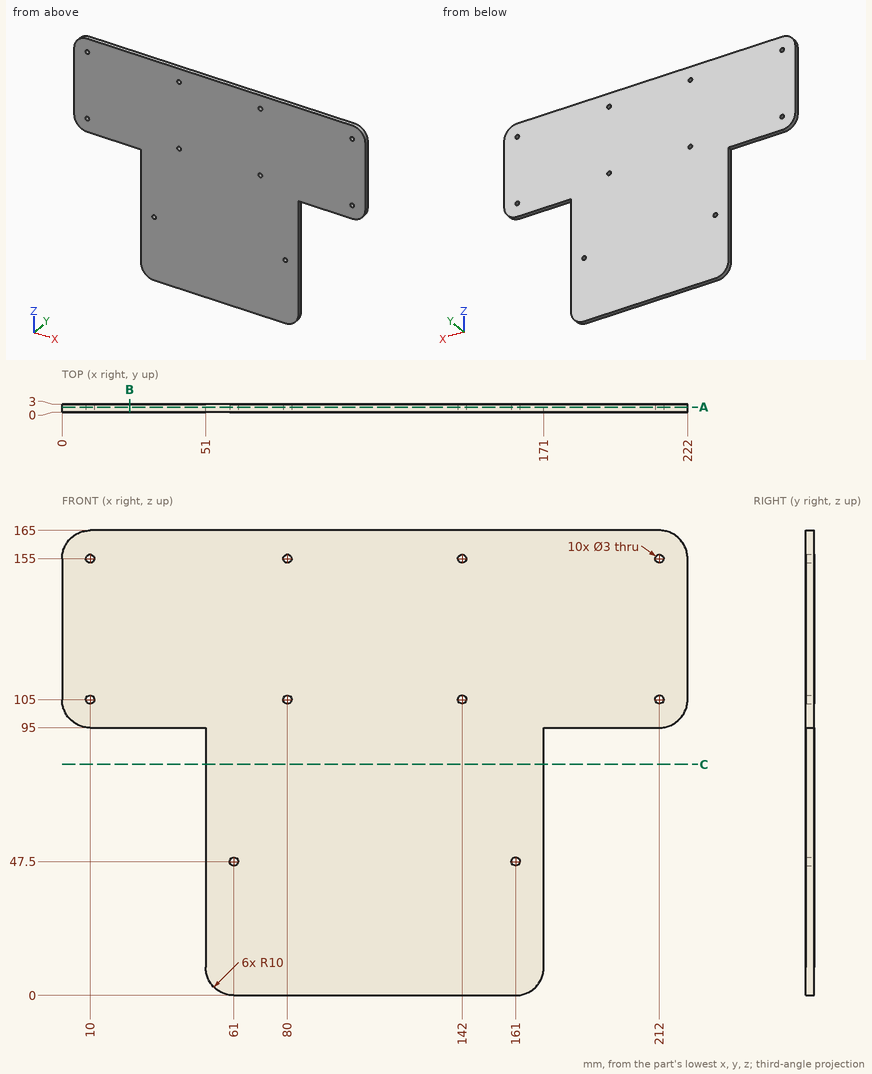
Input: dimensioned drawing with shaded views. Units: mm. Origin: part minimum x, y, z. Give positions to 0.01 mm unless a question says otherwise; leave off trailing zeros. Order: outer loops, then holes, each group sorted by start corner. A loop starts at its lowest first (then second) coordinate and runs counter-clockwise, first axis right, second up. Notation, with made-up numbers: (65, 45) -> (94, 45) arc R24 ccw to (94, 66) -> close; hole circle Ø4 at (22.5, -13.5). An arc over 180 degrees is marked (long way). Use a Markdown table: item, result.
1) Section query A-A, the plane y = 1.9. Count the separate pieces of the cut face and the enclosed holes in it, then the cut area to 3 significant figures.
Answer list:
| item | result |
|---|---|
| separate pieces | 1 |
| enclosed holes | 10 |
| area | 26,700 mm² |
2) Section query B-B, the plane x = 24. Return the cut outline in (y, z).
Answer list:
| item | result |
|---|---|
| outline | (0, 95) -> (3, 95) -> (3, 165) -> (0, 165) -> close |
3) Section query C-C, the plane z = 82. Return the cut outline in (x, y), then the cut area to 3 significant figures.
Answer list:
| item | result |
|---|---|
| outline | (51, 0) -> (171, 0) -> (171, 3) -> (51, 3) -> close |
| area | 360 mm² |
4) Contact query for flat-ended pins moving along their axis: P1, Ø1.5, axis at y = 1, z = 44.5, coming from the +X side; P2, Ø1, axis at y = 1, z = 98, coming from the -X side; P3, Ø0.9, axis at y = 1, z = 72, coming from the -X side. Output: stop coordinate, or through.
Answer list:
| item | result |
|---|---|
| P1 | x = 171 |
| P2 | x = 2.4 |
| P3 | x = 51 |
5) Ray query, line 1 along X through (y, z) = (1.9, 105); line 2 along Z through (x, y) = (212, 2.2); line 3 along Z through (x, y) = (142, 2). Return the intervals inside material, ascending. Write a range as [from, to].
Answer list:
| item | result |
|---|---|
| line 1 | [0, 8.5], [11.5, 78.5], [81.5, 140.5], [143.5, 210.5], [213.5, 222] |
| line 2 | [95, 103.5], [106.5, 153.5], [156.5, 165] |
| line 3 | [0, 103.5], [106.5, 153.5], [156.5, 165] |
